The model under review builds one solid part; all positions refer to its coordinate system, in mm. Face numbers are marked on the shaded views. Coordinates: 2 decimals unless noted, no trailing zeros. Order: outer loops, then holes, each group sorted by start corner. A loop starts at its lowest first (then second) coordinate and runs counter-clockwise, first axis right, second up.
Autodesk Fusion 360 part; units mm, degrees
sketch "Sketch1" plane through (0, 0, 0) normal (0, 0, 1) x (1, 0, 0)
  line L0 (0, 0) -> (20, 0)
  line L1 (20, 8) -> (0, 8)
  line L2 (0, 8) -> (0, 0)
  line L3 (20, 0) -> (25.7446, 4)
  line L4 (25.7446, 4) -> (20, 8)
  circle A0 centre (8, 4) radius 3.5
  dimension "d1" = 20
  dimension "d2" = 8
  dimension "d3" = 7
  dimension "d4" = 7
  dimension "d9" = 8
extrude "Extrude1" add sketch "Sketch1" along normal blind 3
extrude "Extrude2" add sketch "Sketch1" along normal blind 20 contours A0
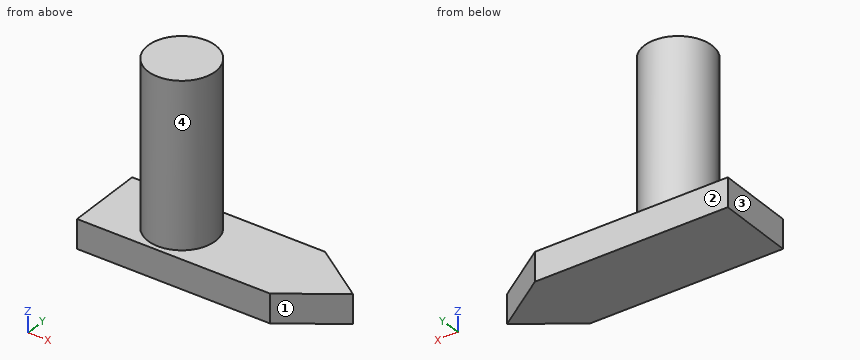
(1) Wall thickness on probe 1 along Z at (x, y) = (4, 7.75); probe 2 along X at (y, z) = (2, 17); probe 3 along X at (y, z) = (5.25, 7.5): over which ranges is each line inside the solid? List them lowest first.
A:
probe 1: z = 0 to 3
probe 2: x = 5.13 to 10.87
probe 3: x = 4.73 to 11.27
(2) For pin 1 Ø1 at (x, y) = (14, 2.5) entering from +Z, flat-tipped, find the tip position at first contact; note if it passes through.
A:
pin 1: stops at z = 3
(3) We need section A-A, the plane x = 8. Write out the cut boundary in (y, z).
A:
outline: (0, 0) - (8, 0) - (8, 3) - (7.5, 3) - (7.5, 20) - (0.5, 20) - (0.5, 3) - (0, 3) - close
(4) We need section C-C, the plane x = 18.75. Write out the cut boundary in (y, z).
A:
outline: (0, 0) - (8, 0) - (8, 3) - (0, 3) - close
(5) We need section B-B, the plane z = 6.75. Write out the cut boundary in (x, y), and give its area (3 significant figures).
A:
outline: circle Ø7 at (8, 4)
area: 38.5 mm2
(6) Draft analysis for pull direction X (two halves, no side actions). For the marked faces 1, 2, 3 and 4, state which applies: released by +X, released by -X, zero draft, split by the parting line, or undercut.
A:
face 1: released by +X
face 2: zero draft
face 3: released by -X
face 4: split by the parting line
